from build123d import *

# Parameters (mm, degrees)
SKETCH2_W           = 47.78
SKETCH2_H           = 3.16
BOSS_EXTRUDE1_DEPTH = 7.81
SKETCH3_R           = 2.455
BOSS_EXTRUDE2_DEPTH = 1.94
SHELL1_T            = -1.6
SKETCH4_R           = 1.495
SKETCH4_R_2         = 0.595
BOSS_EXTRUDE3_DEPTH = 1.36


with BuildPart() as part:
    # Sketch2 → Boss-Extrude1 (new body)
    with BuildSketch(Plane.XY):
        Rectangle(SKETCH2_W, SKETCH2_H)
    extrude(amount=-BOSS_EXTRUDE1_DEPTH)

    # Sketch3 → Boss-Extrude2 (add)
    with BuildSketch(Plane(origin=(0, 1.58, 0), x_dir=(1, 0, 0), z_dir=(0, 1, 0))):
        with Locations(Location((-19.925, 3.905, 0), (0, 0, 270))):
            Circle(SKETCH3_R)
        with Locations(Location((-11.945, 3.905, 0), (0, 0, 270))):
            Circle(SKETCH3_R)
        with Locations(Location((-3.965, 3.905, 0), (0, 0, 270))):
            Circle(SKETCH3_R)
        with Locations(Location((3.965, 3.905, 0), (0, 0, 90))):
            Circle(SKETCH3_R)
        with Locations(Location((11.945, 3.905, 0), (0, 0, 90))):
            Circle(SKETCH3_R)
        with Locations(Location((19.925, 3.905, 0), (0, 0, 90))):
            Circle(SKETCH3_R)
    extrude(amount=BOSS_EXTRUDE2_DEPTH)

    # Shell1
    shell1_openings = [part.faces().sort_by_distance(p)[0] for p in [
        (0, -1.58, -3.905),
    ]]
    offset(amount=SHELL1_T, openings=shell1_openings, kind=Kind.INTERSECTION)

    # Sketch4 → Boss-Extrude3 (add)
    # profile 1 of 5: a face of its own
    with BuildSketch(Plane.XZ.offset(0.02)):
        with Locations(Location((-15.935, -3.905, 0), (0, 0, 90))):
            Circle(SKETCH4_R)
        with Locations(Location((-15.935, -3.905, 0), (0, 0, 270))):
            Circle(SKETCH4_R_2, mode=Mode.SUBTRACT)
    # profile 2 of 5: a face of its own
    with BuildSketch(Plane.XZ.offset(0.02)):
        with Locations(Location((-7.955, -3.905, 0), (0, 0, 90))):
            Circle(SKETCH4_R)
        with Locations(Location((-7.955, -3.905, 0), (0, 0, 270))):
            Circle(SKETCH4_R_2, mode=Mode.SUBTRACT)
    # profile 3 of 5: a face of its own
    with BuildSketch(Plane.XZ.offset(0.02)):
        with Locations(Location((0, -3.905, 0), (0, 0, 90))):
            Circle(SKETCH4_R)
        with Locations(Location((0, -3.905, 0), (0, 0, 270))):
            Circle(SKETCH4_R_2, mode=Mode.SUBTRACT)
    # profile 4 of 5: a face of its own
    with BuildSketch(Plane.XZ.offset(0.02)):
        with Locations(Location((7.955, -3.905, 0), (0, 0, 90))):
            Circle(SKETCH4_R)
        with Locations(Location((7.955, -3.905, 0), (0, 0, 90))):
            Circle(SKETCH4_R_2, mode=Mode.SUBTRACT)
    # profile 5 of 5: a face of its own
    with BuildSketch(Plane.XZ.offset(0.02)):
        with Locations(Location((15.935, -3.905, 0), (0, 0, 90))):
            Circle(SKETCH4_R)
        with Locations(Location((15.935, -3.905, 0), (0, 0, 90))):
            Circle(SKETCH4_R_2, mode=Mode.SUBTRACT)
    extrude(amount=BOSS_EXTRUDE3_DEPTH)


solid = part.part
Here's how the part is built. I have some questions about the finished solid (model axes, mm). A direction names the side the tool comes from. Round coordinates to 2 decimals unless told otherwise and drop trailing zeros. Write each loop counter-clockwise with the first axis right and the second up, starting at its lowest first coordinate (ties: lowest second). Pieces come first, ordered by that corner, then holes.
1. Suppose I cut it at B-B (x = 0). List the corners of the cut face in (y, z) for me.
2. Suppose I cut it at D-D (x = 11.5). List the corners of the cut face in (y, z) for me, and give its area (3 significant figures).
3. Suppose I cut it at C-C (z = -0.5). List the corners of the cut face in (x, y) for me.
4. Suppose I cut it at A-A (y = -0.9). State how many separate pieces and enclosed holes the cut face has, and give its area (3 significant figures).
5. If we mould it in two halves opening along Z, with no side actions, what happens to faces 4 (the cylindrical face through (12.78, 0.94, -3.72)), 5 (the flat face through (0, 0, -7.81)), 6 (the cylindrical face through (-21.42, 2.54, -5.85)), 7 (the flat face through (-12, 3.52, -4))? For each: released by +Z, released by -Z, zero draft, split by the parting line, or undercut.
6. For faces 1 (the cylindrical face through (-3.857, 2.536, -6.358)), 2 (the flat face through (-23.89, 0, -4)), 3 (the flat face through (0, -1, -6.21)), which set-ups out of +Z, -Z, +X, -X, +Y, -Y let a thin tool reach every point of the face, with its end or its side?
7. I need wall thicknesses on L1, parallel to Z at x = -8, y = -1.3; L2, parallel to Z at x = -5, y = -0.35; L3, parallel to Z at x = -1, y = -0.9. Which ranges of each line are inside material? Lowest first, please.
8. Will these pins go through, and if not, where does the flat tip stop? pin 1 Ø1.3 at (x, z) = (-8, -4) entering from -Y; pin 2 Ø1 at (x, z) = (-15.935, -3.905) entering from +Y; pin 3 Ø0.9 at (x, z) = (-12, -4) entering from -Y.
Answer sheet:
1. outline: (-1.58, -7.81) - (1.58, -7.81) - (1.58, 0) - (-1.58, 0) - (-1.58, -1.6) - (-0.02, -1.6) - (-0.02, -2.41) - (-1.38, -2.41) - (-1.38, -3.31) - (-0.02, -3.31) - (-0.02, -4.5) - (-1.38, -4.5) - (-1.38, -5.4) - (-0.02, -5.4) - (-0.02, -6.21) - (-1.58, -6.21) - close
2. outline: (-1.58, -7.81) - (1.58, -7.81) - (1.58, -6.32) - (3.52, -6.32) - (3.52, -1.49) - (1.58, -1.49) - (1.58, 0) - (-1.58, 0) - (-1.58, -1.6) - (-0.02, -1.6) - (-0.02, -3.17) - (1.92, -3.17) - (1.92, -4.64) - (-0.02, -4.64) - (-0.02, -6.21) - (-1.58, -6.21) - close
2. area: 24.0 mm2
3. outline: (-23.89, -1.58) - (23.89, -1.58) - (23.89, 1.58) - (-23.89, 1.58) - close
4. separate pieces: 6
4. enclosed holes: 6
4. area: 197 mm2
5. face 4: undercut
5. face 5: released by -Z
5. face 6: split by the parting line
5. face 7: zero draft
6. face 1: +Y
6. face 2: +Z, -Z, -X, +Y, -Y
6. face 3: -Y
7. L1: z = -7.81 to -6.21, -5.4 to -4.5, -3.31 to -2.41, -1.6 to 0
7. L2: z = -7.81 to -6.21, -1.6 to 0
7. L3: z = -7.81 to -6.21, -5.02 to -2.79, -1.6 to 0
8. pin 1: stops at y = -1.38
8. pin 2: stops at y = 1.58
8. pin 3: stops at y = 1.92
